Autodesk Inventor part; units mm, degrees
ref_plane "Plano de trabajo1" through (-105, 0, 15) normal (0, 1, 0) x (1, 0, 0)
ref_plane "YZ Plane" through (0, 0, 0) normal (1, 0, 0) x (0, 1, 0)
ref_plane "XZ Plane" through (0, 0, 0) normal (0, 1, 0) x (-1, 0, 0)
sketch "Boceto1" plane through (0, 0, 0) normal (0, 0, 1) x (1, 0, 0)
  circle A0 centre (0, 0) radius 20
  line L0 (0, 0) -> (0, 37.5) construction
  line L1 (0, 0) -> (-32.476, -18.75) construction
  line L2 (0, 0) -> (32.476, -18.75) construction
  circle A1 centre (0, 0) radius 27.5 construction
  circle A2 centre (0, 32.5) radius 2.5
  circle A3 centre (-28.1458, -16.25) radius 2.5
  circle A4 centre (28.1458, -16.25) radius 2.5
  line L3 (0, 37.5) -> (0, 105) construction
  line L4 (-54.0833, 90) -> (54.0833, 90)
  line L5 (54.0833, -90) -> (-54.0833, -90)
  arc A5 (-54.0833, 90) -> (-54.0833, -90) centre (0, 0) ccw
  arc A6 (54.0833, -90) -> (54.0833, 90) centre (0, 0) ccw
  point P0 (0, 27.5)
  dimension "d2" = 55
  dimension "d1" = 40
  dimension "d3" = 10
  dimension "d4" = 120
  dimension "d5" = 120
  dimension "d6" = 120
  dimension "d7" = 5
  dimension "d8" = 5
  dimension "d11" = 360
  dimension "d13" = 90
  dimension "d16" = 360
  dimension "d18" = 105
extrude "Extrusión1" add sketch "Boceto1" along normal blind 15
sketch "Boceto2" plane through (-54.0833, 90, 0) normal (0, 1, 0) x (1, 0, 0)
  line L0 (54.0833, 0) -> (54.0833, -15) construction
  line L1 (108.1665, -15) -> (0, -15) construction
  line L2 (0, 0) -> (0, -15) construction
  line L3 (0, -7.5) -> (108.1665, -7.5) construction
  line L4 (108.1665, 0) -> (108.1665, -15) construction
  circle A0 centre (54.0833, -7.5) radius 5
  dimension "d21" = 10
extrude "Extrusión2" cut sketch "Boceto2" against normal blind 20
ref_plane "Plano de trabajo1" through (-105, 0, 15) normal (0, 1, 0) x (1, 0, 0)
mirror "Simetría1" about plane through (-105, 0, 15) normal (0, 1, 0) of "Extrusión2"
properties part number "Tapa cvt"
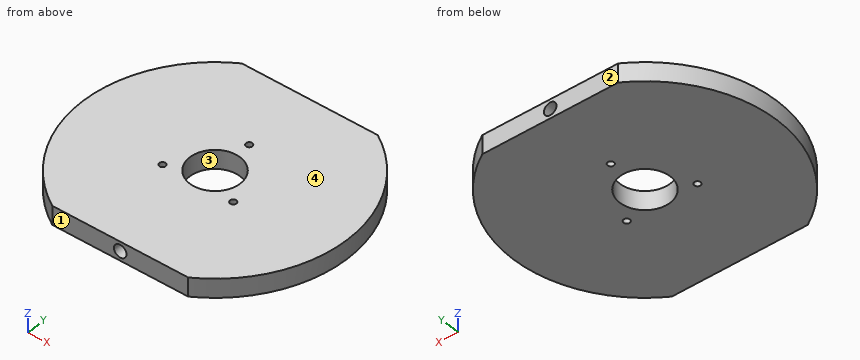
Geometry: final body of the model. Coordinates: model frame, mm. Face numbers are marked on the shaded views. Round coordinates to 2 decimals unless told otherwise and drop trailing zeros. Order: outer loops, then holes, each group sorted by start corner. A loop starts at its lowest first (then second) coordinate and runs counter-clockwise, first axis right, second up.
Q1. Section D-D, the plane x = 81. Output: boundary loops of the cut face in (y, z).
Result sheet:
outline: (-66.81, 0) - (66.81, 0) - (66.81, 15) - (-66.81, 15) - close
Q2. Mould query, pull axis Y, two halves, no side actions, for the marked faces 1, 2, 3 and 4. Classes: released by +Y, released by -Y, zero draft, split by the parting line, or undercut.
Result sheet:
face 1: released by -Y
face 2: released by +Y
face 3: undercut
face 4: zero draft
Q3. Material intervals for probe 1 along Y at (x, z) = (0, 8.5); probe 2 along Y at (x, z) = (-0.5, 1.25); probe 3 along Z at (x, y) = (0, 84.5), sorted ascending.
Result sheet:
probe 1: y = -70 to -20, 20 to 30, 35 to 70
probe 2: y = -90 to -19.99, 19.99 to 30.05, 34.95 to 90
probe 3: z = 0 to 2.5, 12.5 to 15
Q4. Pin query (flat end, axial travel): pin 1 (9 mm diameter, centred on x = 0, z = 7.5, fed in from -Y); pin 2 (6 mm diameter, centred on y = -18, z = 6, fed in from -X); pin 3 (1.5 mm diameter, centred on y = -7, z = 4, fed in from -X); pin 4 (24 mm diameter, centred on x = 0, y = 0, fed in from +Z). Return the tip coordinate at first contact, or that it passes through.
Result sheet:
pin 1: stops at y = -70
pin 2: stops at x = -103.92
pin 3: stops at x = -104.81
pin 4: passes through
Q5. Section B-B, the plane x = 0. Output: boundary loops of the cut face in (y, z), and give its area (4 significant figures).
Result sheet:
outline: (-90, 0) - (-20, 0) - (-20, 15) - (-90, 15) - (-90, 12.5) - (-70, 12.5) - (-70, 2.5) - (-90, 2.5) - close; (20, 0) - (30, 0) - (30, 15) - (20, 15) - close; (35, 0) - (90, 0) - (90, 2.5) - (70, 2.5) - (70, 12.5) - (90, 12.5) - (90, 15) - (35, 15) - close
area: 1,625 mm2
Q6. Section A-A, the plane y = -4. Output: boundary loops of the cut face in (x, z), and give its area (3 significant figures).
Result sheet:
outline: (-104.92, 0) - (-19.6, 0) - (-19.6, 15) - (-104.92, 15) - close; (19.6, 0) - (104.92, 0) - (104.92, 15) - (19.6, 15) - close
area: 2,560 mm2
Q7. Section C-C, the plane y = 32.5. Output: boundary loops of the cut face in (x, z), and give its area (3 significant figures).
Result sheet:
outline: (-99.84, 0) - (-2.5, 0) - (-2.5, 15) - (-99.84, 15) - close; (2.5, 0) - (99.84, 0) - (99.84, 15) - (2.5, 15) - close
area: 2,920 mm2
